The model under review builds one solid part; all positions refer to its coordinate system, in mm. Coordinates: 2 decimals unless noted, no trailing zeros. Order: outer loops, then holes, each group sorted by start corner. A loop starts at its lowest first (then second) coordinate and runs counter-clockwise, first axis right, second up. Notation, with made-up numbers: M -3.5,2.25 L 35.5,2.25 A14 ccw 35.5,24.25 Z; hole C 54,34.25 d10. An arc over 180 degrees is marked long. One line per item, written item: value.
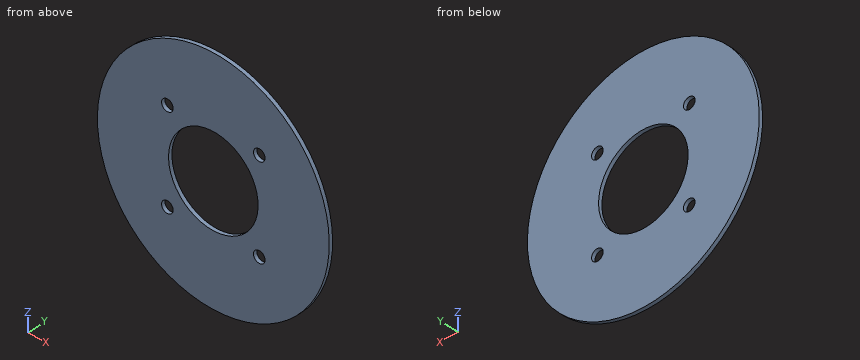
```python
from build123d import *

# Parameters (mm, degrees)
SKETCH_1_R          = 29
EXTRUDE_1_DEPTH     = 0.9
SKETCH_2_R          = 1.45
SKETCH_2_R_2        = 11.2
CUT_EXTRUDE_1_DEPTH = 0.9


with BuildPart() as part:
    # 草图1 → 凸台-拉伸1 (new body)
    with BuildSketch(Plane.XZ.offset(-604.003613165)):
        with Locations(Location((0, 0, 0), (0, 0, 270))):
            Circle(SKETCH_1_R)
    extrude(amount=EXTRUDE_1_DEPTH)

    # 草图2 → 切除-拉伸1 (cut)
    with BuildSketch(Plane.XZ.offset(-603.103613165)):
        with Locations(Location((11.5, -11.5, 0), (0, 0, 270))):
            Circle(SKETCH_2_R)
        with Locations(Location((-11.5, -11.5, 0), (0, 0, 270))):
            Circle(SKETCH_2_R)
        with Locations(Location((11.5, 11.5, 0), (0, 0, 270))):
            Circle(SKETCH_2_R)
        with Locations(Location((-11.5, 11.5, 0), (0, 0, 270))):
            Circle(SKETCH_2_R)
        with Locations(Location((0, 0, 0), (0, 0, 270))):
            Circle(SKETCH_2_R_2)
    extrude(amount=-CUT_EXTRUDE_1_DEPTH, mode=Mode.SUBTRACT)


solid = part.part
```
(1) We need section A-A, the plane x = 0. State the section outline as (y, z) points, plus the area to 3 significant figures.
Geometry results:
outline: M 603.1,-29 L 604,-29 L 604,-11.2 L 603.1,-11.2 Z; M 603.1,11.2 L 604,11.2 L 604,29 L 603.1,29 Z
area: 32.0 mm2
(2) We need section C-C, the plane z = -2. State the section outline as (x, y) points.
Geometry results:
outline: M -28.93,603.1 L -11.02,603.1 L -11.02,604 L -28.93,604 Z; M 11.02,603.1 L 28.93,603.1 L 28.93,604 L 11.02,604 Z
(3) We need section D-D, the plane z = -12. State the section outline as (x, y) points.
Geometry results:
outline: M -26.4,603.1 L -12.86,603.1 L -12.86,604 L -26.4,604 Z; M -10.14,603.1 L 10.14,603.1 L 10.14,604 L -10.14,604 Z; M 12.86,603.1 L 26.4,603.1 L 26.4,604 L 12.86,604 Z
(4) For L1, parallel to X at y = 603.4, z = 11.5; L2, parallel to Z at x = 12.5, y = 603.2; L3, parallel to X at y = 603.3, z = 0, list the stretches that pass through material, from the lowest coordinate up.
Geometry results:
L1: x = -26.62 to -12.95, -10.05 to 10.05, 12.95 to 26.62
L2: z = -26.17 to -12.55, -10.45 to 10.45, 12.55 to 26.17
L3: x = -29 to -11.2, 11.2 to 29
(5) We need section B-B, the plane y = 603.85. State the section outline as (x, z) points.
Geometry results:
outline: C 0,0 d58; hole C -11.5,-11.5 d2.9; hole C -11.5,11.5 d2.9; hole C 0,0 d22.4; hole C 11.5,-11.5 d2.9; hole C 11.5,11.5 d2.9
